The listing builds one solid part. Answer for the finished solid, in the listing's coordinates (mm). A direction names the side the tool comes from. Coordinates: 2 decimals unless noted, no trailing zeros. Order: outer loops, then holes, each group sorted by start corner. A loop starts at its lowest first (then second) coordinate and runs counter-clockwise, first axis right, second up.
Autodesk Inventor part; units mm, degrees
ref_plane "YZ Plane" through (0, 0, 0) normal (1, 0, 0) x (0, 1, 0)
ref_plane "XZ Plane" through (0, 0, 0) normal (0, 1, 0) x (-1, 0, 0)
ref_plane "XY Plane" through (0, 0, 0) normal (0, 0, 1) x (1, 0, 0)
sketch "スケッチ1" plane through (0, 0, 0) normal (0, 0, 1) x (1, 0, 0)
  line L0 (-10, -7.5) -> (10, -7.5)
  line L1 (10, -7.5) -> (10, 7.5)
  line L2 (10, 7.5) -> (-10, 7.5)
  line L3 (-10, 7.5) -> (-10, -7.5)
  line L4 (-10, -7.5) -> (10, 7.5) construction
  line L5 (10, -7.5) -> (-10, 7.5) construction
  point P0 (0, 0)
  dimension "d0" = 20
  dimension "d1" = 15
extrude "押し出し1" add sketch "スケッチ1" along normal mid plane 3
sketch "スケッチ2" plane through (0, 0, 1.5) normal (0, 0, 1) x (1, 0, 0)
  line L0 (10, -7.5) -> (10, 7.5)
  line L1 (-10, -3.05) -> (10, -3.05)
  line L2 (10, -3.05) -> (10, 3.05)
  line L3 (10, 3.05) -> (-10, 3.05)
  line L4 (-10, 3.05) -> (-10, -3.05)
  line L5 (-10, -3.05) -> (10, 3.05) construction
  line L6 (10, -3.05) -> (-10, 3.05) construction
  point P0 (0, 0)
  dimension "d4" = 6.1
extrude "押し出し2" cut sketch "スケッチ2" against normal blind 0.6
sketch "スケッチ3" plane through (0, 0, 0.9) normal (0, 0, 1) x (1, 0, 0)
  line L0 (-1.35, 0) -> (1.35, 0) construction
  line L1 (-1.35, -1.35) -> (1.35, -1.35)
  line L2 (1.35, 1.35) -> (-1.35, 1.35)
  arc A0 (-1.35, 1.35) -> (-1.35, -1.35) centre (-1.35, 0) ccw
  arc A1 (1.35, -1.35) -> (1.35, 1.35) centre (1.35, 0) ccw
  point P0 (0, 0)
  point P1 (2.7, 0)
  point P2 (-2.7, 0)
  dimension "d7" = 2.7
  dimension "d8" = 5.4
extrude "押し出し3" add sketch "スケッチ3" along normal blind 0.6
sketch "スケッチ4" plane through (0, 0, 0.9) normal (0, 0, 1) x (1, 0, 0)
  line L0 (1.35, -1.35) -> (-1.35, -1.35)
  arc A0 (-1.35, 1.35) -> (-1.35, -1.35) centre (-1.35, 0) ccw
  line L1 (-1.35, 1.35) -> (1.35, 1.35)
  arc A1 (1.35, -1.35) -> (1.35, 1.35) centre (1.35, 0) ccw
  line L2 (10, -3.05) -> (-10, -3.05)
  line L3 (10, 3.05) -> (10, -3.05)
  line L4 (-10, 3.05) -> (10, 3.05)
  line L5 (-10, -3.05) -> (-10, 3.05)
  line L6 (-10, 3.05) -> (10, 3.05)
  line L7 (-6.8, 3.05) -> (-6.8, -3.05)
  arc A2 (-1.35, 1.35) -> (-1.35, -1.35) centre (-1.35, 0) ccw
  point P0 (0, 0)
  point P1 (-2.7, 0)
  dimension "d11" = 4.1
extrude "押し出し4" add sketch "スケッチ4" along normal blind 0.6 contours L2 L5 L4 L7
sketch "スケッチ5" plane through (0, 0, 1.5) normal (0, 0, 1) x (1, 0, 0)
  line L0 (0, 0) -> (2.6024, 0)
  point P0 (-7.5, 5.5)
  point P1 (8, 5.5)
  point P2 (-7.5, -5.5)
  point P3 (8, -5.5)
  dimension "d14" = 5.5
  dimension "d15" = 5.5
  dimension "d16" = 8
  dimension "d17" = 7.5
hole "穴1" at (-7.5, 5.5, 1.5) at (8, 5.5, 1.5) at (-7.5, -5.5, 1.5) at (8, -5.5, 1.5) direction (0, 0, -1) diameter 1.567 end through all
properties part number "cutter_holder"
1) Consider L1, parallel to Y at x = 8, z = 0.8; L2, parallel to X at y = 5.5, z = -0.25; L3, parallel to Y at x = 0.75, z = 1.3. Determine where each line is inside the solid, lowest interval first.
2) Each of these flat-tipped pins is pushed along its axis until it touches: P1, Ø2.5, axis at x = -7.5, y = 5.5, coming from the -Z side; P2, Ø0.5, axis at y = -1, z = 1.5, coming from the +X side. Where does it stop, or does it pass through?
3) Section D-D (x = 4) is taken. Give the vertices of the cut face in (y, z).
4) Section A-A (z = -0.85) is taken. Give the vertices of the cut face in (x, y).
5) Determine the mould class of faces 1 (the face through (-10, 0, 0)), 2 (the face through (0, 0, 1.5)), 3 (the face through (-7.2, 4.776, -0.021)), 4 (the face through (8.695, -5.862, -0.021)) for opening direction X: released by +X, released by -X, zero draft, split by the parting line, or undercut.
6) Section C-C (y = 5.5) is taken. Give the vertices of the cut face in (x, z).
7) A tool of negligible diameter and unlimited length cuts with its end or side. For faces 5 (the face through (2.7, 0, 1.2)), 6 (the face through (-0.1, 3.4, 1.5)), 7 (the face through (-2.7, 0, 1.2)), from which of +Z, -Z, +X, -X, +Y, -Y can it reach the whole face along a straight path? Write none if from no direction.
8) Section B-B (x = 8) is taken. Give the vertices of the cut face in (y, z), then the cut area to 3 significant figures.
Filled sheet:
1. L1: y = -7.5 to -6.28, -4.72 to 4.72, 6.28 to 7.5
1. L2: x = -10 to -8.28, -6.72 to 7.22, 8.78 to 10
1. L3: y = -7.5 to -3.05, -1.35 to 1.35, 3.05 to 7.5
2. P1: stops at z = -1.5
2. P2: stops at x = 2.47
3. outline: (-7.5, -1.5) - (7.5, -1.5) - (7.5, 1.5) - (3.05, 1.5) - (3.05, 0.9) - (-3.05, 0.9) - (-3.05, 1.5) - (-7.5, 1.5) - close
4. outline: (-10, -7.5) - (10, -7.5) - (10, 7.5) - (-10, 7.5) - close; hole circle Ø1.57 at (-7.5, -5.5); hole circle Ø1.57 at (-7.5, 5.5); hole circle Ø1.57 at (8, -5.5); hole circle Ø1.57 at (8, 5.5)
5. face 1: released by -X
5. face 2: zero draft
5. face 3: undercut
5. face 4: undercut
6. outline: (-10, -1.5) - (-8.28, -1.5) - (-8.28, 1.5) - (-10, 1.5) - close; (-6.72, -1.5) - (7.22, -1.5) - (7.22, 1.5) - (-6.72, 1.5) - close; (8.78, -1.5) - (10, -1.5) - (10, 1.5) - (8.78, 1.5) - close
7. face 5: +Z, +X
7. face 6: +Z, +X, -X, +Y, -Y
7. face 7: +Z
8. outline: (-7.5, -1.5) - (-6.28, -1.5) - (-6.28, 1.5) - (-7.5, 1.5) - close; (-4.72, -1.5) - (4.72, -1.5) - (4.72, 1.5) - (3.05, 1.5) - (3.05, 0.9) - (-3.05, 0.9) - (-3.05, 1.5) - (-4.72, 1.5) - close; (6.28, -1.5) - (7.5, -1.5) - (7.5, 1.5) - (6.28, 1.5) - close
8. area: 31.9 mm2
